Here's the drawing with two shaded views (mm, measured from the low corner). I have some questions. A direction names the side the tool comes from. Give positions to 0.01 mm unless a question says otherwise; leave off trailing zeros. Loops run counter-clockwise (first coordinate to the right, second up) from the corner with the lowest first, then second, coordinate; pieces in that order, holes last. Notation, with made-up numbers: M -12.5,-27 L 8.5,-27 A22 cw 8.5,-12 Z; hole C 50.25,75.25 d4. An arc over 180 degrees is marked long. Use a Markdown table: item, result. Add a question column.
1) Suppose I cut it at C-C on x = 66.25. List the corners of the cut face in (y, z) for me.
2) Will these pins go through, and if not, where does the flat tip stop? pin 1 Ø1.5 at (x, z) = (47.5, 3.5) entering from -Y; pin 2 Ø5 at (x, y) = (66.25, 23.7) entering from -Z.
3) Suppose I cut it at A-A on y = 13.5. List the corners of the cut face in (x, z) for me, and give its area (3 significant figures).
4) If I drill on line 1 along Y through (x, z) = (66.25, 3.6); line 2 along X through (y, z) = (10.5, 1.3); line 3 along X through (y, z) = (2.5, 3.9), over which ranges is the centre line in solid material (lowest first)? Write a range as [from, to].
5) Suppose I cut it at B-B on y = 23.7. List the corners of the cut face in (x, z) for me.
6) Suppose I cut it at D-D on z = 4.15. List the corners of the cut face in (x, y) for me.
7) Which directions (+Z, -Z, +X, -X, +Y, -Y) give clear straight access to the entire face, cutting with the end or side of a thin tool? Please do the marked faces 1 and 2.
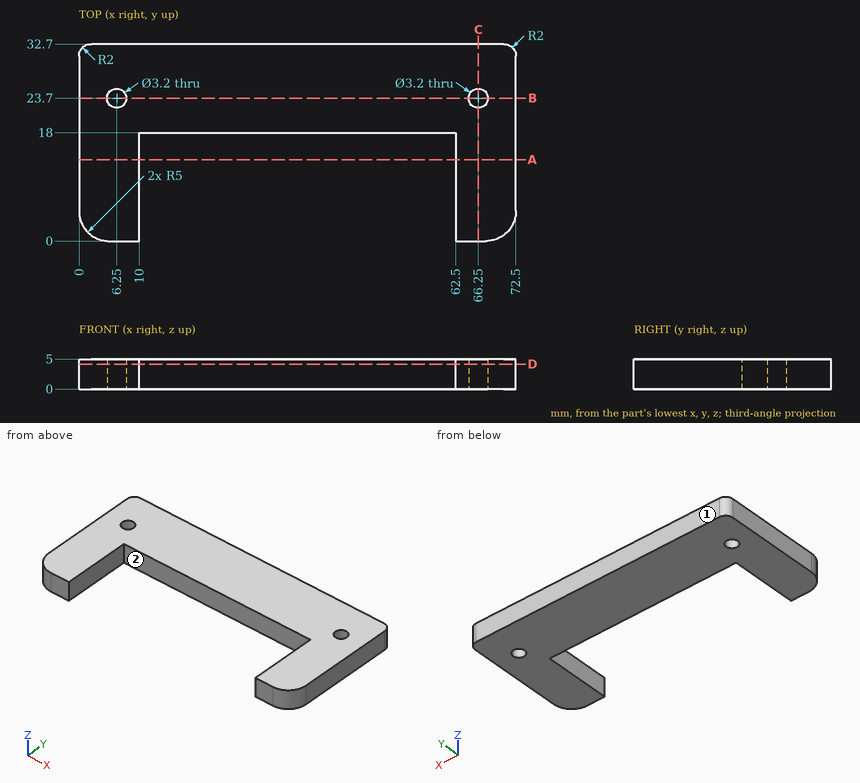
Answer block:
| question | item | result |
|---|---|---|
| 1 | outline | M 0,0 L 22.1,0 L 22.1,5 L 0,5 Z; M 25.3,0 L 32.7,0 L 32.7,5 L 25.3,5 Z |
| 2 | pin 1 | stops at y = 18 |
| 2 | pin 2 | stops at z = 0 |
| 3 | outline | M 0,0 L 10,0 L 10,5 L 0,5 Z; M 62.5,0 L 72.5,0 L 72.5,5 L 62.5,5 Z |
| 3 | area | 100 mm^2 |
| 4 | line 1 | y = [0, 22.1], [25.3, 32.7] |
| 4 | line 2 | x = [0, 10], [62.5, 72.5] |
| 4 | line 3 | x = [0.67, 10], [62.5, 71.83] |
| 5 | outline | M 0,0 L 4.65,0 L 4.65,5 L 0,5 Z; M 7.85,0 L 64.65,0 L 64.65,5 L 7.85,5 Z; M 67.85,0 L 72.5,0 L 72.5,5 L 67.85,5 Z |
| 6 | outline | M 0,5 A5 ccw 5,0 L 10,0 L 10,18 L 62.5,18 L 62.5,0 L 67.5,0 A5 ccw 72.5,5 L 72.5,30.7 A2 ccw 70.5,32.7 L 2,32.7 A2 ccw 0,30.7 Z; hole C 6.25,23.7 d3.2; hole C 66.25,23.7 d3.2 |
| 7 | face 1 | +Z, -Z, +X, -X, +Y |
| 7 | face 2 | +Z, -Z, -Y |
